Autodesk Inventor part; units mm, degrees
ref_plane "YZ Plane" through (0, 0, 0) normal (1, 0, 0) x (0, 1, 0)
ref_plane "XZ Plane" through (0, 0, 0) normal (0, 1, 0) x (-1, 0, 0)
ref_plane "XY Plane" through (0, 0, 0) normal (0, 0, 1) x (1, 0, 0)
sketch "Sketch1" plane through (0, 0, 0) normal (0, 0, 1) x (1, 0, 0)
  line L0 (0, 0) -> (92, 0)
  line L1 (92, 0) -> (92, 20)
  line L2 (92, 20) -> (0, 20)
  line L3 (0, 20) -> (0, 0)
  dimension "d0" = 92
  dimension "d1" = 20
extrude "Extrusion1" add sketch "Sketch1" along normal blind 3
sketch "Sketch2" plane through (0, 0, 3) normal (0, 0, 1) x (1, 0, 0)
  line L0 (0, 0) -> (92, 0)
  line L1 (92, 0) -> (92, 20)
  line L2 (92, 20) -> (0, 20)
  line L3 (0, 20) -> (0, 0)
  circle A0 centre (31, 10) radius 2.1
  circle A1 centre (61, 10) radius 2.1
  dimension "d5" = 4.2
  dimension "d6" = 31
  dimension "d7" = 10
  dimension "d8" = 10
  dimension "d9" = 31
  dimension "d10" = 4.2
extrude "Extrusion2" cut sketch "Sketch2" against normal up to next contours A0 | A1
sketch "Sketch3" plane through (0, 0, 3) normal (0, 0, 1) x (1, 0, 0)
  line L0 (92, 0) -> (92, 20)
  line L1 (0, 0) -> (92, 0)
  line L2 (92, 0) -> (92, 3)
  line L3 (92, 3) -> (0, 3)
  line L4 (0, 3) -> (0, 0)
  dimension "d13" = 3
extrude "Extrusion3" add sketch "Sketch3" along normal blind 30
sketch "Sketch4" plane through (0, 3, 3) normal (0, 1, 0) x (1, 0, 0)
  circle A0 centre (20, -15) radius 5
  line L0 (0, 0) -> (92, 0)
  line L1 (0, 0) -> (0, -30)
  line L2 (92, -30) -> (0, -30)
  line L3 (92, 0) -> (92, -30)
  point P0 (0, 3)
  dimension "d16" = 20
  dimension "d17" = 15
  dimension "d18" = 10
extrude "Extrusion4" cut sketch "Sketch4" against normal blind 30 contours A0
properties part number "EE_Base-Rod-Rev2"
The model under review builds one solid part; all positions refer to its coordinate system, in mm. A direction names the side the tool comes from. Round coordinates to 2 decimals unless told otherwise and drop trailing zeros. Loops run counter-clockwise (first coordinate to the right, second up) from the corner with the lowest first, then second, coordinate; pieces in that order, holes last. Notation, with made-up numbers: (86, 39.5) - (119, 39.5) arc R26 ccw to (119, 62.5) - close; hole circle Ø6 at (-31.75, 62). An arc over 180 degrees is marked (long way). Write each question's results on one line, items separated by ' | '. Start each with the question number.
Q1. Draft analysis for pull direction Y (two halves, no side actions). For faces 1 (the flat face through (45, 2, 33)), 2 (the flat face through (47, 20, 1)), 3 (the cylindrical face through (28.9, 10.09, 1.52)), state which applies: pulls with the +Y half, pulls with the -Y half, needs draft (parallel to the pull), parting line crosses it, or undercut.
Q2. Take a section at B-B on y = 10. Give the boundary of the cut face in (x, z).
Q3. Take a section at A-A on x = 20. Give the boundary of the cut face in (y, z), plus the area to 3 significant figures.
Q4. Take a section at D-D on x = 31. Give the boundary of the cut face in (y, z), plus the area to 3 significant figures.
Q5. Tool access review of faces 4 (the flat face through (45, 0, 16)), 5 (the flat face through (45, 12, 3)): name each direction out of +Z, -Z, +X, -X, +Y, -Y from which nothing blocks a thin tool from reaching the whole face with its end or side.
Q6. Take a section at C-C on z = 18. Give the boundary of the cut face in (x, y), plus the area to 3 significant figures.
Q7. Insertion check: P1, Ø16, axis at x = 20, z = 18, coming from the -Y side; P2, Ø9, axis at x = 28, z = 23.5, coming from the +Y side; P3, Ø3, axis at x = 34.5, y = 14, coming from the +Z side. Each pin has a flat end and moves straight along its axis. Give the tip position at first contact, or say it passes through.
Q8. Wall thickness on line 1 along Y through (x, z) = (61, 0.8); line 2 along X through (y, z) = (2, 18); line 3 along Y through (x, z) = (12, 25.5): over which ranges is each line inside the solid? List them lowest first. Write a range as [from, to].
Data:
1) face 1: needs draft | face 2: pulls with the +Y half | face 3: undercut
2) outline: (0, 0) - (28.9, 0) - (28.9, 3) - (0, 3) - close; (33.1, 0) - (58.9, 0) - (58.9, 3) - (33.1, 3) - close; (63.1, 0) - (92, 0) - (92, 3) - (63.1, 3) - close
3) outline: (0, 0) - (20, 0) - (20, 3) - (3, 3) - (3, 13) - (0, 13) - close; (0, 23) - (3, 23) - (3, 33) - (0, 33) - close | area: 120 mm²
4) outline: (0, 0) - (7.9, 0) - (7.9, 3) - (3, 3) - (3, 33) - (0, 33) - close; (12.1, 0) - (20, 0) - (20, 3) - (12.1, 3) - close | area: 137 mm²
5) face 4: +Z, -Z, +X, -X, -Y | face 5: +Z, +X, -X, +Y
6) outline: (0, 0) - (15, 0) - (15, 3) - (0, 3) - close; (25, 0) - (92, 0) - (92, 3) - (25, 3) - close | area: 246 mm²
7) P1: stops at y = 0 | P2: stops at y = 3 | P3: stops at z = 3
8) line 1: y = [0, 7.9], [12.1, 20] | line 2: x = [0, 15], [25, 92] | line 3: y = [0, 3]
